Design review of the part built by this model. Coordinates are the model's own, in mm. Coordinates: 2 decimals unless noted, no trailing zeros. Loops run counter-clockwise (first coordinate to the right, second up) from the corner with the lowest first, then second, coordinate; pieces in that order, holes last. Notation, with made-up numbers: (-33.5, 70) -> (19.5, 70) arc R29 cw to (19.5, 90) -> close; hole circle Ø3 at (47, 59.5). An arc over 180 degrees is marked (long way). One line per item, written item: value. Start each with the question number.
1. Draft analysis for pull direction Z (two halves, no side actions). For faces 1 (the cylindrical face through (2.46, 8.31, -0.01)), 2 (the flat face through (13, 0, 3)), state which applies: pulls with the +Z half, pulls with the -Z half, needs draft (parallel to the pull), parting line crosses it, or undercut.
2. For probe 1 along Z at (x, y) = (1.5, -6.75); probe 2 along Z at (x, y) = (4.75, -7.75); probe 3 along Y at (x, z) = (10, 0), list the stretches that pass through material, from the lowest coordinate up.
3. Add section B-B on z = 0. Write out the cut boundary in (x, y).
4. Insertion check: pin 1 (2 mm diameter, centred on x = 6.5, z = -4.5, fed in from +Y); pin 2 (2 mm diameter, centred on y = 9.5, z = -8.5, fed in from -X); pin 3 (6 mm diameter, centred on x = 4, z = -8.5, fed in from +Y); pin 4 (4 mm diameter, centred on y = 0, z = 0, fed in from -X) (3 decimals). Each pin has a flat end and moves straight along its axis. Give the tip position at first contact, or say it passes through.
5. Add section C-C on z = 5.75. Write out the cut boundary in (x, y) (3 decimals).
6. Add section D-D on x = 5.5. Write out the cut boundary in (y, z), plus the area to 3 significant figures.
7. Add section A-A on y = 0. Write out the cut boundary in (x, z) (1 decimal).
```python
from build123d import *

# Parameters (mm, degrees)
METRIC_SPUR_GEAR_1_75M_12T_20PA_5FW_OU_R  = 2.5
METRIC_SPUR_GEAR_1_75M_12T_20PA_5FW_DEPTH = 5
SKETCH2_R                                 = 7.5
SKETCH2_R_2                               = 2.5
BOSS_EXTRUDE1_DEPTH                       = 13
SKETCH3_R                                 = 1.375
CUT_EXTRUDE1_DEPTH                        = 13
CUT_EXTRUDE2_DEPTH                        = 22.281227002
CUT_EXTRUDE2_DEPTH_BACK                   = 22.281227002
SKETCH4_R                                 = 2.6


# Read off the part's stored shape, not the designer's step: Metric - Spur gear 1.75M 12T 20PA 5FW ---S12N75H50L5N
with BuildPart() as part:
    # Metric - Spur gear 1.75M 12T 20PA 5FW ou → Metric - Spur gear 1.75M 12T 20PA 5FW (new body)
    with BuildSketch(Plane.YZ):
        with BuildLine():
            ThreePointArc((8.893362097, 8.424405653), (8.66205807, 8.66205807), (8.424405653, 8.893362097))
            ThreePointArc((8.424405653, 8.893362097), (6.40252905, 8.232977147), (4.963463004, 6.666713378))
            ThreePointArc((4.963463004, 6.666713378), (4.15575, 7.197970144), (3.291811643, 7.631841741))
            ThreePointArc((3.291811643, 7.631841741), (3.928702834, 9.661241379), (3.489674675, 11.742430356))
            ThreePointArc((3.489674675, 11.742430356), (3.170533302, 11.832591372), (2.849068258, 11.914080328))
            ThreePointArc((2.849068258, 11.914080328), (1.428264232, 10.331231883), (0.965128363, 8.255274647))
            ThreePointArc((0.965128363, 8.255274647), (0, 8.3115), (-0.965128363, 8.255274647))
            ThreePointArc((-0.965128363, 8.255274647), (-1.428264232, 10.331231883), (-2.849068258, 11.914080328))
            ThreePointArc((-2.849068258, 11.914080328), (-3.170533302, 11.832591372), (-3.489674675, 11.742430356))
            ThreePointArc((-3.489674675, 11.742430356), (-3.928702834, 9.661241379), (-3.291811643, 7.631841741))
            ThreePointArc((-3.291811643, 7.631841741), (-4.15575, 7.197970144), (-4.963463004, 6.666713378))
            ThreePointArc((-4.963463004, 6.666713378), (-6.40252905, 8.232977147), (-8.424405653, 8.893362097))
            ThreePointArc((-8.424405653, 8.893362097), (-8.66205807, 8.66205807), (-8.893362097, 8.424405653))
            ThreePointArc((-8.893362097, 8.424405653), (-8.232977147, 6.40252905), (-6.666713378, 4.963463004))
            ThreePointArc((-6.666713378, 4.963463004), (-7.197970144, 4.15575), (-7.631841741, 3.291811643))
            ThreePointArc((-7.631841741, 3.291811643), (-9.661241379, 3.928702834), (-11.742430356, 3.489674675))
            ThreePointArc((-11.742430356, 3.489674675), (-11.832591372, 3.170533302), (-11.914080328, 2.849068258))
            ThreePointArc((-11.914080328, 2.849068258), (-10.331231883, 1.428264232), (-8.255274647, 0.965128363))
            ThreePointArc((-8.255274647, 0.965128363), (-8.3115, 0), (-8.255274647, -0.965128363))
            ThreePointArc((-8.255274647, -0.965128363), (-10.331231883, -1.428264232), (-11.914080328, -2.849068258))
            ThreePointArc((-11.914080328, -2.849068258), (-11.832591372, -3.170533302), (-11.742430356, -3.489674675))
            ThreePointArc((-11.742430356, -3.489674675), (-9.661241379, -3.928702834), (-7.631841741, -3.291811643))
            ThreePointArc((-7.631841741, -3.291811643), (-7.197970144, -4.15575), (-6.666713378, -4.963463004))
            ThreePointArc((-6.666713378, -4.963463004), (-8.232977147, -6.40252905), (-8.893362097, -8.424405653))
            ThreePointArc((-8.893362097, -8.424405653), (-8.66205807, -8.66205807), (-8.424405653, -8.893362097))
            ThreePointArc((-8.424405653, -8.893362097), (-6.40252905, -8.232977147), (-4.963463004, -6.666713378))
            ThreePointArc((-4.963463004, -6.666713378), (-4.15575, -7.197970144), (-3.291811643, -7.631841741))
            ThreePointArc((-3.291811643, -7.631841741), (-3.928702834, -9.661241379), (-3.489674675, -11.742430356))
            ThreePointArc((-3.489674675, -11.742430356), (-3.170533302, -11.832591372), (-2.849068258, -11.914080328))
            ThreePointArc((-2.849068258, -11.914080328), (-1.428264232, -10.331231883), (-0.965128363, -8.255274647))
            ThreePointArc((-0.965128363, -8.255274647), (0, -8.3115), (0.965128363, -8.255274647))
            ThreePointArc((0.965128363, -8.255274647), (1.428264232, -10.331231883), (2.849068258, -11.914080328))
            ThreePointArc((2.849068258, -11.914080328), (3.170533302, -11.832591372), (3.489674675, -11.742430356))
            ThreePointArc((3.489674675, -11.742430356), (3.928702834, -9.661241379), (3.291811643, -7.631841741))
            ThreePointArc((3.291811643, -7.631841741), (4.15575, -7.197970144), (4.963463004, -6.666713378))
            ThreePointArc((4.963463004, -6.666713378), (6.40252905, -8.232977147), (8.424405653, -8.893362097))
            ThreePointArc((8.424405653, -8.893362097), (8.66205807, -8.66205807), (8.893362097, -8.424405653))
            ThreePointArc((8.893362097, -8.424405653), (8.232977147, -6.40252905), (6.666713378, -4.963463004))
            ThreePointArc((6.666713378, -4.963463004), (7.197970144, -4.15575), (7.631841741, -3.291811643))
            ThreePointArc((7.631841741, -3.291811643), (9.661241379, -3.928702834), (11.742430356, -3.489674675))
            ThreePointArc((11.742430356, -3.489674675), (11.832591372, -3.170533302), (11.914080328, -2.849068258))
            ThreePointArc((11.914080328, -2.849068258), (10.331231883, -1.428264232), (8.255274647, -0.965128363))
            ThreePointArc((8.255274647, -0.965128363), (8.3115, 0), (8.255274647, 0.965128363))
            ThreePointArc((8.255274647, 0.965128363), (10.331231883, 1.428264232), (11.914080328, 2.849068258))
            ThreePointArc((11.914080328, 2.849068258), (11.832591372, 3.170533302), (11.742430356, 3.489674675))
            ThreePointArc((11.742430356, 3.489674675), (9.661241379, 3.928702834), (7.631841741, 3.291811643))
            ThreePointArc((7.631841741, 3.291811643), (7.197970144, 4.15575), (6.666713378, 4.963463004))
            ThreePointArc((6.666713378, 4.963463004), (8.232977147, 6.40252905), (8.893362097, 8.424405653))
        make_face()
        Circle(METRIC_SPUR_GEAR_1_75M_12T_20PA_5FW_OU_R, mode=Mode.SUBTRACT)
    extrude(amount=METRIC_SPUR_GEAR_1_75M_12T_20PA_5FW_DEPTH)

    # Sketch2 → Boss-Extrude1 (add)
    with BuildSketch(Plane(origin=(0, 0, 0), x_dir=(0, 0, -1), z_dir=(1, 0, 0))):
        with Locations(Location((0, 0, 0), (0, 0, 180))):
            Circle(SKETCH2_R)
        Circle(SKETCH2_R_2, mode=Mode.SUBTRACT)
    extrude(amount=BOSS_EXTRUDE1_DEPTH)

    # Sketch3 → Cut-Extrude1 (cut)
    with BuildSketch(Plane.XY):
        with Locations((10, 0)):
            Circle(SKETCH3_R)
    extrude(amount=CUT_EXTRUDE1_DEPTH, mode=Mode.SUBTRACT)

    # Sketch4 → Cut-Extrude2 (cut, two sides: drawn at the far end of the back side and taken through both)
    with BuildSketch(Plane(origin=(0, 0, 0), x_dir=(0, 0, -1), z_dir=(1, 0, 0)).offset(-CUT_EXTRUDE2_DEPTH_BACK)):
        Circle(SKETCH4_R)
    extrude(amount=CUT_EXTRUDE2_DEPTH + CUT_EXTRUDE2_DEPTH_BACK, mode=Mode.SUBTRACT)


solid = part.part
```
Worked answers:
1. face 1: undercut
1. face 2: needs draft
2. probe 1: z = -8.43 to -5.01, -4.85 to 4.85, 5.01 to 8.43
2. probe 2: z = -8.8 to -5.79, -3.36 to 3.36, 5.79 to 8.8
2. probe 3: y = -7.5 to -2.6, 2.6 to 7.5
3. outline: (0, -8.31) -> (5, -8.31) -> (5, -7.5) -> (13, -7.5) -> (13, -2.6) -> (0, -2.6) -> close; (0, 2.6) -> (13, 2.6) -> (13, 7.5) -> (5, 7.5) -> (5, 8.31) -> (0, 8.31) -> close
4. pin 1: stops at y = 6.63
4. pin 2: stops at x = 0
4. pin 3: stops at y = 8.89
4. pin 4: passes through
5. outline: (0, -7.715) -> (5, -7.715) -> (5, -4.815) -> (13, -4.815) -> (13, 4.815) -> (5, 4.815) -> (5, 7.715) -> (0, 7.715) -> close; hole circle Ø2.75 at (10, 0)
6. outline: circle Ø15 at (0, 0); hole circle Ø5.2 at (0, 0)
6. area: 155 mm²
7. outline: (0, -8.3) -> (5, -8.3) -> (5, -7.5) -> (13, -7.5) -> (13, -2.6) -> (0, -2.6) -> close; (0, 2.6) -> (8.6, 2.6) -> (8.6, 7.5) -> (5, 7.5) -> (5, 8.3) -> (0, 8.3) -> close; (11.4, 2.6) -> (13, 2.6) -> (13, 7.5) -> (11.4, 7.5) -> close
